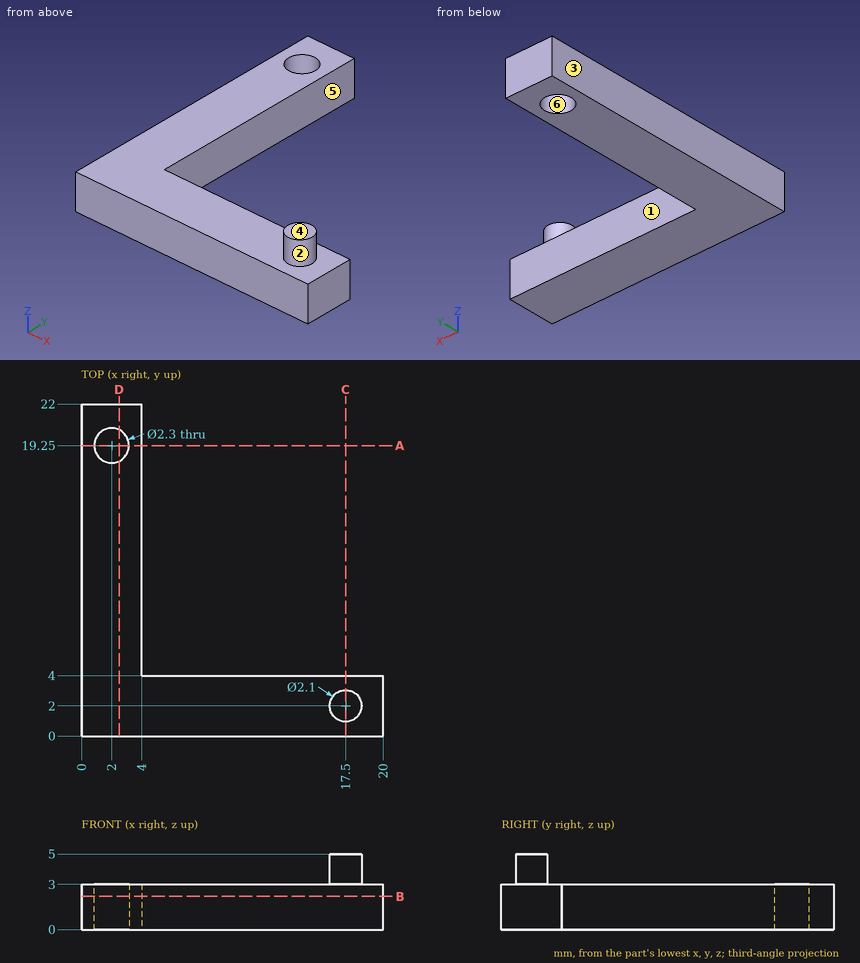
Geometry check sheet. Reference: drawing and pictorial views, mm from the part's lowest x, y, z. A direction names the side the tool comes from. Coordinates: 2 decimals unless noted, no trailing zeros. Write each loop counter-clockwise with the first axis right and the second up, starting at its lowest first coordinate (ties: lowest second). Pieces come first, ordered by that corner, then holes. Notation, with made-up numbers: M 58,1 L 83,1 A23 cw 83,39 Z; hole C 7,68.5 d7. An arc over 180 degrees is marked long. Use one line per item in the form item = value.
Item 1: Sectioned sample at D-D, the plane x = 2.5. Record the cut outline in (y, z), and give its area (3 significant figures).
Answer below:
outline = M 0,0 L 18.21,0 L 18.21,3 L 0,3 Z; M 20.29,0 L 22,0 L 22,3 L 20.29,3 Z
area = 59.8 mm^2
Item 2: Release check for a two-part mould opening along X. For the marked faces 4, 5 and 6 record: pulls with the +X half, pulls with the -X half, needs draft (parallel to the pull), parting line crosses it, or undercut.
Answer below:
face_4 = needs draft
face_5 = pulls with the +X half
face_6 = undercut
Item 3: Sectioned sample at C-C, the plane x = 17.5. Record the cut outline in (y, z), and give its area (3 significant figures).
Answer below:
outline = M 0,0 L 4,0 L 4,3 L 3.05,3 L 3.05,5 L 0.95,5 L 0.95,3 L 0,3 Z
area = 16.2 mm^2
Item 4: Material ranges on L1, parallel to Y at x = 2, z = 2.15; L2, parallel to X at y = 21, z = 2.8; L3, parallel to Z at x = 18.75, y = 3.5, recorded low to high. Write a range as from..to.
Answer below:
L1 = 0..18.1, 20.4..22
L2 = 0..4
L3 = 0..3
Item 5: Sectioned sample at B-B, the plane z = 2.2. Record the cut outline in (x, y).
Answer below:
outline = M 0,0 L 20,0 L 20,4 L 4,4 L 4,22 L 0,22 Z; hole C 2,19.25 d2.3
Item 6: Gauge pin test, flat ends, axial feed: pin 1 Ø1.5 at (y, z) = (12.5, 1.5) entering from +X; pin 2 Ø1.5 at (x, z) = (8.5, 1.5) entering from +Y. Record the tip position at first contact, or that the pin passes through.
Answer below:
pin_1 = 4
pin_2 = 4
Item 7: Set-up check for the marked faces 1, 2 and 3: record each of +Z, -Z, +X, -X, +Y, -Y from which the full face is reachable in a straight line by a thin tool's end or side.
Answer below:
face_1 = +Z, -Z, +X, +Y
face_2 = +Z
face_3 = +Z, -Z, -X, +Y, -Y
Item 8: Sectioned sample at A-A, the plane y = 19.25. Record the cut outline in (x, z), and give its area (3 significant figures).
Answer below:
outline = M 0,0 L 0.85,0 L 0.85,3 L 0,3 Z; M 3.15,0 L 4,0 L 4,3 L 3.15,3 Z
area = 5.10 mm^2
